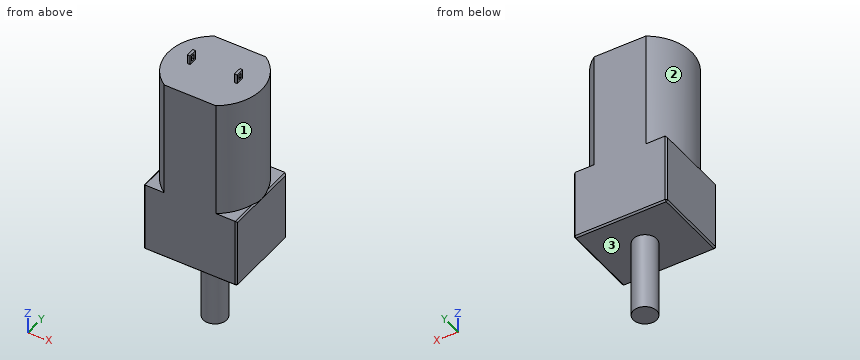
from build123d import *

# Parameters (mm, degrees)
SKETCH_1_W          = 12
SKETCH_1_H          = 10
EXTRUDE_2_DEPTH     = 9
EXTRUDE_4_DEPTH     = 15
CHAMFER_4_SIZE      = 0.2
SKETCH_4_W          = 0.352238381
SKETCH_4_H          = 1.084523436
EXTRUDE_5_DEPTH     = 1.2
SKETCH_5_W          = 0.65
SKETCH_5_H          = 0.45
CUT_EXTRUDE_1_DEPTH = 28.29282553
SKETCH_6_R          = 1.5
EXTRUDE_6_DEPTH     = 10


with BuildPart() as part:
    # 草图1 → 凸台-拉伸2 (new body)
    with BuildSketch(Plane.XY):
        Rectangle(SKETCH_1_W, SKETCH_1_H)
    extrude(amount=EXTRUDE_2_DEPTH)

    # 草图2 → 凸台-拉伸4 (add)
    with BuildSketch(Plane.XY.offset(9)):
        with BuildLine():
            Line((-3.31662479, 5), (3.31662479, 5))
            ThreePointArc((3.31662479, 5), (6, 0), (3.31662479, -5))
            Line((3.31662479, -5), (-3.31662479, -5))
            ThreePointArc((-3.31662479, -5), (-6, 0), (-3.31662479, 5))
        make_face()
    extrude(amount=EXTRUDE_4_DEPTH)

    # 倒角4
    # the kernel refuses this chamfer: 0.2 mm, written as the material it takes off along each edge
    with BuildSketch(Plane(origin=(-5.866666667, -4.866666667, 0.133333333), x_dir=(-0.7071067811865491, 0.707106781186546, 0), z_dir=(-0.577350269189624, -0.5773502691896265, -0.5773502691896268)), Plane(origin=(5.866666667, 4.866666667, 0.133333333), x_dir=(-0.7071067811865478, -3.1401849173675483e-15, -0.7071067811865472), z_dir=(0.577350269189624, 0.5773502691896265, -0.577350269189627))) as chamfer_4_piece_1:
        Polygon((-0.141421356, -0.081649658), (0.141421356, -0.081649658), (0, 0.163299316), align=None)
    extrude(amount=0.254034118, mode=Mode.SUBTRACT)
    with BuildSketch(Plane(origin=(5.866666667, -4.866666667, 0.133333333), x_dir=(0.707106781186546, 0.7071067811865491, 0), z_dir=(0.5773502691896265, -0.577350269189624, -0.577350269189627)), Plane(origin=(-5.866666667, 4.866666667, 0.133333333), x_dir=(0.7071067811865478, 0, -0.7071067811865472), z_dir=(-0.5773502691896265, 0.577350269189624, -0.5773502691896268))) as chamfer_4_piece_2:
        Polygon((-0.141421356, 0.081649658), (0.141421356, 0.081649658), (0, -0.163299316), align=None)
    extrude(amount=0.254034118, mode=Mode.SUBTRACT)
    with BuildSketch(Plane(origin=(-6, 5.514336598, 9), x_dir=(-0.02749587661058742, 0, -0.9996219169112966), z_dir=(0, -1, 0))) as chamfer_4_piece_3_section:
        Polygon((CHAMFER_4_SIZE * 0.999621916911, CHAMFER_4_SIZE * 0.0274958766106), (-CHAMFER_4_SIZE * 0.0274958766106, CHAMFER_4_SIZE * 0.999621916911), (0, 0), align=None)
    chamfer_4_piece_3 = extrude(amount=5.514336598, mode=Mode.PRIVATE)
    chamfer_4_piece_3 = chamfer_4_piece_3 - Plane(origin=(0, 0, 8.93146509), x_dir=(-0.5527707983925667, -0.8333333333333334, 0), z_dir=(0, 0, -1)) * Cylinder(6, 12, mode=Mode.PRIVATE)
    add(chamfer_4_piece_3, mode=Mode.SUBTRACT)
    with BuildSketch(Plane(origin=(6, 0, 9), x_dir=(0.02749587661058742, 0, -0.9996219169112966), z_dir=(0, 1, 0))) as chamfer_4_piece_4_section:
        Polygon((CHAMFER_4_SIZE * 0.999621916911, CHAMFER_4_SIZE * 0.0274958766106), (-CHAMFER_4_SIZE * 0.0274958766106, CHAMFER_4_SIZE * 0.999621916911), (0, 0), align=None)
    chamfer_4_piece_4 = extrude(amount=5.514336598, mode=Mode.PRIVATE)
    chamfer_4_piece_4 = chamfer_4_piece_4 - Plane(origin=(0, 0, 8.931465093), x_dir=(0.5527707983925666, 0.8333333333333334, 0), z_dir=(0, 0, -1)) * Cylinder(6, 12, mode=Mode.PRIVATE)
    add(chamfer_4_piece_4, mode=Mode.SUBTRACT)
    with BuildSketch(Plane(origin=(-6, 0, 9), x_dir=(-0.02749587661058742, 0, -0.9996219169112966), z_dir=(0, -1, 0))) as chamfer_4_piece_5_section:
        Polygon((CHAMFER_4_SIZE * 0.999621916911, CHAMFER_4_SIZE * 0.0274958766106), (-CHAMFER_4_SIZE * 0.0274958766106, CHAMFER_4_SIZE * 0.999621916911), (0, 0), align=None)
    chamfer_4_piece_5 = extrude(amount=5.514336598, mode=Mode.PRIVATE)
    chamfer_4_piece_5 = chamfer_4_piece_5 - Plane(origin=(0, 0, 8.931465093), x_dir=(-0.5527707983925667, -0.8333333333333334, 0), z_dir=(0, 0, -1)) * Cylinder(6, 12, mode=Mode.PRIVATE)
    add(chamfer_4_piece_5, mode=Mode.SUBTRACT)
    with BuildSketch(Plane(origin=(6, -5.514336598, 9), x_dir=(0.02749587661058742, 0, -0.9996219169112966), z_dir=(0, 1, 0))) as chamfer_4_piece_6_section:
        Polygon((CHAMFER_4_SIZE * 0.999621916911, CHAMFER_4_SIZE * 0.0274958766106), (-CHAMFER_4_SIZE * 0.0274958766106, CHAMFER_4_SIZE * 0.999621916911), (0, 0), align=None)
    chamfer_4_piece_6 = extrude(amount=5.514336598, mode=Mode.PRIVATE)
    chamfer_4_piece_6 = chamfer_4_piece_6 - Plane(origin=(0, 0, 8.93146509), x_dir=(0.5527707983925666, 0.8333333333333334, 0), z_dir=(0, 0, -1)) * Cylinder(6, 12, mode=Mode.PRIVATE)
    add(chamfer_4_piece_6, mode=Mode.SUBTRACT)
    with BuildSketch(Plane(origin=(-6.514336598, -5, 0), x_dir=(0, -0.02749587661058735, 0.9996219169112966), z_dir=(1, 0, 0))) as chamfer_4_piece_7:
        Polygon((CHAMFER_4_SIZE * 0.999621916911, -CHAMFER_4_SIZE * 0.0274958766106), (-CHAMFER_4_SIZE * 0.0274958766106, -CHAMFER_4_SIZE * 0.999621916911), (0, 0), align=None)
    extrude(amount=13.028673195, mode=Mode.SUBTRACT)
    with BuildSketch(Plane(origin=(-6, 5.514336598, 0), x_dir=(-0.02749587661058735, 0, 0.9996219169112966), z_dir=(0, -1, 0)), Plane(origin=(6, -5.514336598, 0), x_dir=(0.02749587661058735, 0, 0.9996219169112966), z_dir=(0, 1, 0))) as chamfer_4_piece_8:
        Polygon((CHAMFER_4_SIZE * 0.999621916911, -CHAMFER_4_SIZE * 0.0274958766106), (-CHAMFER_4_SIZE * 0.0274958766106, -CHAMFER_4_SIZE * 0.999621916911), (0, 0), align=None)
    extrude(amount=11.028673195, mode=Mode.SUBTRACT)
    with BuildSketch(Plane(origin=(6.514336598, 5, 0), x_dir=(0, -0.9996219169112968, -0.027495876610586313), z_dir=(-1, 0, 0))) as chamfer_4_piece_9:
        Polygon((CHAMFER_4_SIZE * 0.999621916911, CHAMFER_4_SIZE * 0.0274958766106), (-CHAMFER_4_SIZE * 0.0274958766106, CHAMFER_4_SIZE * 0.999621916911), (0, 0), align=None)
    extrude(amount=13.028673195, mode=Mode.SUBTRACT)
    with BuildSketch(Plane(origin=(6, -5, -0.514336598), x_dir=(-0.9996219169112966, -0.02749587661058742, 0), z_dir=(0, 0, 1)), Plane(origin=(6, 5, -0.514336598), x_dir=(0.02749587661058742, -0.9996219169112966, 0), z_dir=(0, 0, 1))) as chamfer_4_piece_10:
        Polygon((CHAMFER_4_SIZE * 0.999621916911, -CHAMFER_4_SIZE * 0.0274958766106), (-CHAMFER_4_SIZE * 0.0274958766106, -CHAMFER_4_SIZE * 0.999621916911), (0, 0), align=None)
    extrude(amount=10.028673195, mode=Mode.SUBTRACT)
    with BuildSketch(Plane(origin=(-6, -5, -0.514336598), x_dir=(0.9996219169112966, -0.027495876610587302, 0), z_dir=(0, 0, 1)), Plane(origin=(-6, 5, -0.514336598), x_dir=(-0.027495876610587302, -0.9996219169112966, 0), z_dir=(0, 0, 1))) as chamfer_4_piece_11:
        Polygon((CHAMFER_4_SIZE * 0.999621916911, CHAMFER_4_SIZE * 0.0274958766106), (-CHAMFER_4_SIZE * 0.0274958766106, CHAMFER_4_SIZE * 0.999621916911), (0, 0), align=None)
    extrude(amount=10.028673195, mode=Mode.SUBTRACT)

    # 草图4 → 凸台-拉伸5 (add)
    with BuildSketch(Plane.XY.offset(24)):
        with Locations((-3.035738681, 0)):
            Rectangle(SKETCH_4_W, SKETCH_4_H)
        with Locations((3.035738681, 0)):
            Rectangle(SKETCH_4_W, SKETCH_4_H)
    extrude(amount=EXTRUDE_5_DEPTH)

    # 草图5 → 切除-拉伸1 (cut, through all)
    with BuildSketch(Plane(origin=(3.211857871, 0, 0), x_dir=(0, 0, -1), z_dir=(1, 0, 0))):
        with Locations((-24.6, 0)):
            Rectangle(SKETCH_5_W, SKETCH_5_H)
    extrude(amount=-CUT_EXTRUDE_1_DEPTH, mode=Mode.SUBTRACT)

    # 草图6 → 凸台-拉伸6 (add)
    with BuildSketch(Plane(origin=(0, 0, 0), x_dir=(-1, 0, 0), z_dir=(0, 0, -1))):
        Circle(SKETCH_6_R)
    extrude(amount=EXTRUDE_6_DEPTH)


solid = part.part
Check sheet for the modelled part. Datum: model origin and axes. Units: mm. Face numbers are marked on the shaded views. A direction names the side the tool comes from. Give positions to 0.01 mm unless a question says otherwise; leave off trailing zeros. Write each loop counter-clockwise with the first axis right and the second up, starting at its lowest first coordinate (ties: lowest second). Pieces come first, ordered by that corner, then holes. Notation, with made-up numbers: (17, 48.5) -> (68, 48.5) arc R21 cw to (68, 87.5) -> close; hole circle Ø1 at (-25.75, 15.25). An arc over 180 degrees is marked (long way). One line per item, written item: value. Start each with the question number.
Item 1: Section check A-A on x = 0. Record the cut outline in (y, z).
Item 2: Material ranges on probe 1 along Z at (x, y) = (-3, 1.5); probe 2 along Z at (x, y) = (-5, 3.75); probe 3 along X at (y, z) = (-1, 17), recorded low to high. Write a range as from..to.
Item 3: Section check C-C on y = 3. Record the cut outline in (x, z).
Item 4: Section check D-D on y = -2.5. Record the cut outline in (x, z), then the cut area to 3 significant figures.
Item 5: Gauge pin test, flat ends, axial feed: pin 1 (4 mm diameter, centred on x = -4, z = 17, fed in from -Y); pin 2 (1.2 mm diameter, centred on y = 0, z = 25, fed in from +X); pin 3 (1.2 mm diameter, centred on x = -4, y = -3, fed in from +Z); pin 4 (0.9 mm diameter, centred on y = 0, z = 24.5, fed in from -X). Record the tip position at first contact, or that the pin passes through.
Item 6: Tool access check on the marked faces 1, 2 and 3. Record the directions out of +Z, -Z, +X, -X, +Y, -Y that give a thin tool (end or side, any length) a straight path to the whole face; none if there is none.
Item 7: Section check B-B on z = 21.5. Record the cut outline in (x, y).
Results list:
1. outline: (-5, 0.2) -> (-4.8, 0) -> (-1.5, 0) -> (-1.5, -10) -> (1.5, -10) -> (1.5, 0) -> (4.8, 0) -> (5, 0.2) -> (5, 24) -> (-5, 24) -> close
2. probe 1: 0..24
2. probe 2: 0..9
2. probe 3: -5.92..5.92
3. outline: (-6, 0.2) -> (-5.8, 0) -> (5.8, 0) -> (6, 0.2) -> (6, 8.8) -> (5.8, 9) -> (5.2, 9) -> (5.2, 24) -> (-5.2, 24) -> (-5.2, 9) -> (-5.8, 9) -> (-6, 8.8) -> close
4. outline: (-6, 0.2) -> (-5.8, 0) -> (5.8, 0) -> (6, 0.2) -> (6, 8.8) -> (5.8, 9) -> (5.45, 9) -> (5.45, 24) -> (-5.45, 24) -> (-5.45, 9) -> (-5.8, 9) -> (-6, 8.8) -> close
4. area: 272 mm²
5. pin 1: y = -5
5. pin 2: x = 3.21
5. pin 3: z = 24
5. pin 4: x = -3.21
6. face 1: +Z, +X
6. face 2: +Z, -X
6. face 3: -Z
7. outline: (-3.32, -5) -> (3.32, -5) arc R6 ccw to (3.32, 5) -> (-3.32, 5) arc R6 ccw to start
